Check sheet for the modelled part. Datum: model origin and axes. Units: mm. A direction names the side the tool comes from. Give positions to 0.01 mm unless a question says otherwise; leave off trailing zeros. Order: outer loops, then holes, each group sorted by start corner. A loop starts at its lowest first (then second) coordinate and runs counter-clockwise, first axis right, second up. Notation, with made-up numbers: M -8,-13 L -2,-13 A16 cw -2,-8 Z; hole C 79.25,-27.5 d4. An arc over 180 degrees is marked long. Answer in a Markdown table with one row per item. Add a question column.
from build123d import *

# Parameters (mm, degrees)
F2_W     = 1.5875
F2_H     = 0.79375
F4_SIZE  = 1.5875
F5_R     = 0.381
F7_D     = 5.1054
F7_DEPTH = 12.7
F7_TIP   = 1.5338169022


with BuildPart() as f1:
    # F0 (on Front) → F1 (revolve)
    with BuildSketch(Plane.XZ):
        Polygon((-114.3, 0), (0, 0), (0, 12.7), (-38.1, 12.7), (-38.1, 20.6375), (-84.1375, 20.6375), (-84.1375, 12.6492), (-101.6, 12.6492), (-114.3, 5.3168515813), align=None)
    revolve(axis=Axis((-57.15, 0, 0), (1, 0, 0)))

    # F2 (on Top) → F3 (revolve, cut)
    with BuildSketch(Plane.XY):
        with Locations((-37.30625, -12.303125)):
            Rectangle(F2_W, F2_H)
    revolve(axis=Axis((-65.0381594896, 0, 0), (-1, 0, 0)), mode=Mode.SUBTRACT)

    # F4
    f4_edges = [f1.edges().sort_by_distance(p)[0] for p in [
        (0, 0, -12.7),
        (-38.1, 0, -20.6375),
        (-84.1375, 0, -20.6375),
    ]]
    chamfer(f4_edges, length=F4_SIZE)

    # F5
    f5_edges = [f1.edges().sort_by_distance(p)[0] for p in [
        (-84.1375, 0, -12.6492),
    ]]
    fillet(f5_edges, radius=F5_R)

    # F7
    with Locations(Plane.YZ):
        with Locations((0, 0)):
            Hole(F7_D / 2, depth=F7_DEPTH)
            with Locations((0, 0, -(F7_DEPTH + F7_TIP / 2))):  # 118° drill point
                Cone(0, F7_D / 2, F7_TIP, mode=Mode.SUBTRACT)


solid = f1.part
Q1. Cross-section at C-C (x = -92). Record the boundary of the cut face in (y, z), and give its area (3 significant figures).
Q2. Tool access check on faces 1 (the cylindrical face through (-93, -4, 12)), 2 (the cylindrical face through (-6.439, -2.435, 0.767)), 3 (the cylindrical face through (-61.419, 20.147, -4.474)). Record the directions out of +Z, -Z, +X, -X, +Y, -Y that give a thin tool (end or side, any length) a straight path to the whole face; none if there is none.
Q3. Go/stop test with flat-tipped pins: pin 1 (3 mm diameter, centred on y = 0, z = -13.5, fed in from -X); pin 2 (12 mm diameter, centred on x = -68.5, y = 8, fed in from -Z); pin 3 (1.5 mm diameter, centred on x = -92.5, z = -7, fed in from +Y). Record where each tip stops, or that it passes through.
Q4. Cross-section at B-B (x = -66). Record the boundary of the cut face in (y, z) (1 decimal), and give its area (3 significant figures).
Q5. Thickness scan on probe 1 along Z at (x, y) = (-7, 0); probe 2 along X at (y, z) = (5, 16). Record the ranges inside material, lowest first.
Q6. Cross-section at A-A (x = -7.5). Record the boundary of the cut face in (y, z).
Q7. Draft check along X on faces 4 (the conical face through (-13.967, 0.41, -0.17)), 5 (the cylindrical face through (-37.3, 9.45, -7.24)), 6 (the conical face through (-112.27, 5.76, 2.99)), 7 (the cylindrical face through (-19.29, 12.4, -2.75)). Enter one of: pulls with the +X half, pulls with the -X half, needs draft (parallel to the pull), parting line crosses it, or undercut.
Values follow:
| question | item | result |
|---|---|---|
| 1 | outline | C 0,0 d25.3 |
| 1 | area | 503 mm² |
| 2 | face 1 | -X |
| 2 | face 2 | +X |
| 2 | face 3 | +X, -X |
| 3 | pin 1 | x = -102.72 |
| 3 | pin 2 | z = -20.54 |
| 3 | pin 3 | y = 11 |
| 4 | outline | C 0,0 d41.3 |
| 4 | area | 1,340 mm² |
| 5 | probe 1 | -12.7 to -2.55, 2.55 to 12.7 |
| 5 | probe 2 | -84.14 to -38.1 |
| 6 | outline | C 0,0 d25.4; hole C 0,0 d5.11 |
| 7 | face 4 | pulls with the +X half |
| 7 | face 5 | undercut |
| 7 | face 6 | pulls with the -X half |
| 7 | face 7 | needs draft |
